from build123d import *

# Parameters (mm, degrees)
F0_W        = 50.8
F0_H        = 50.8
F1_DEPTH    = 546.1
F2_T        = -2.54
F3_T1_DEPTH = 506.0659394114
F5_D        = 41.275


# Not quite as in the source:
# - a fillet or chamfer that OpenCascade refuses, or shapes differently, is made with other operations: its cross-section is extruded or revolved along the edge and cut away or added


with BuildPart() as f1:
    # F0 (on Front) → F1 (new body, symmetric)
    with BuildSketch(Plane.XZ):
        Rectangle(F0_W, F0_H)
    extrude(amount=F1_DEPTH, both=True)

    # F2
    f2_openings = [f1.faces().sort_by_distance(p)[0] for p in [
        (0, -546.1, 0),
        (0, 546.1, 0),
    ]]
    offset(amount=F2_T, openings=f2_openings)

    # F3: chamfer of 50.8 x 87.9881810245 on 1 edges, made by hand

    # F3_s2 → F3_t1 (cut)
    with BuildSketch(Plane.XY.offset(-253.0329697057)):
        Polygon((25.4, 458.1118189755), (-25.4, 546.1), (25.4, 546.1), align=None)
    extrude(amount=F3_T1_DEPTH, mode=Mode.SUBTRACT)

    # F5 (through all)
    with Locations(Plane.XY.offset(25.4)):
        with Locations((0, -520.7)):
            Hole(F5_D / 2)


solid = f1.part
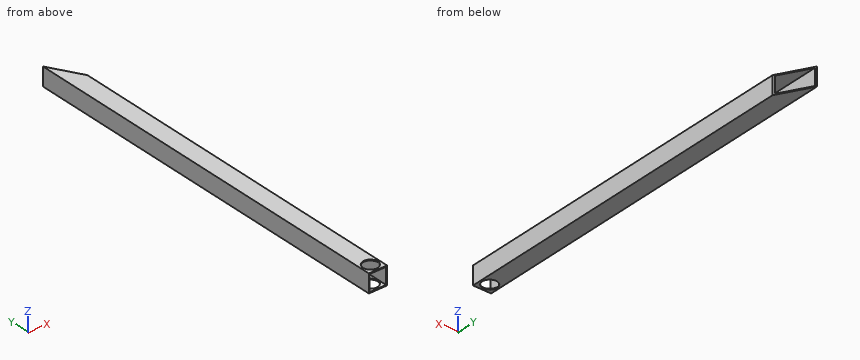
Geometry check sheet. Reference: the model listing, model coordinates, mm. Coordinates: 2 decimals unless noted, no trailing zeros. Order: outer loops, then holes, each group sorted by start corner. A loop starts at its lowest first (then second) coordinate and runs counter-clockwise, first axis right, second up. Notation, with made-up numbers: (-37, -6) - (-23, -6) arc R8 cw to (-23, 0) - close; hole circle Ø5 at (5, -13.5). An arc over 180 degrees is marked (long way). One line per item, written item: value.
(1) Sectioned sample at D-D (y = -156.5). Enter the section's corners in (x, z).
Data:
outline: (-25.4, -25.4) - (25.4, -25.4) - (25.4, 25.4) - (-25.4, 25.4) - close; hole (-22.86, -22.86) - (22.86, -22.86) - (22.86, 22.86) - (-22.86, 22.86) - close
(2) Sectioned sample at A-A (y = -520.7). Enter the section's corners in (x, z).
Data:
outline: (-25.4, -25.4) - (-20.64, -25.4) - (-20.64, -22.86) - (-22.86, -22.86) - (-22.86, 22.86) - (-20.64, 22.86) - (-20.64, 25.4) - (-25.4, 25.4) - close; (20.64, -25.4) - (25.4, -25.4) - (25.4, 25.4) - (20.64, 25.4) - (20.64, 22.86) - (22.86, 22.86) - (22.86, -22.86) - (20.64, -22.86) - close
(3) Sectioned sample at B-B (z = 5). Enter the section's corners in (x, y).
Data:
outline: (-25.4, -546.1) - (-22.86, -546.1) - (-22.86, 541.7) - (-25.4, 546.1) - close; (22.86, -546.1) - (25.4, -546.1) - (25.4, 458.11) - (22.86, 462.51) - close
(4) Sectioned sample at C-C (x = 0). Enter the section's corners in (y, z).
Data:
outline: (-546.1, -25.4) - (-541.34, -25.4) - (-541.34, -22.86) - (-546.1, -22.86) - close; (-546.1, 22.86) - (-541.34, 22.86) - (-541.34, 25.4) - (-546.1, 25.4) - close; (-500.06, -25.4) - (502.11, -25.4) - (502.11, -22.86) - (-500.06, -22.86) - close; (-500.06, 22.86) - (502.11, 22.86) - (502.11, 25.4) - (-500.06, 25.4) - close
(5) Thickness scan on probe 1 along Z at (x, y) = (-3, -147.5); probe 2 along X at (y, z) = (488.5, 2.5). Record the ranges inside material, lowest first. Write a range as from..to.
Data:
probe 1: z = -25.4..-22.86, 22.86..25.4
probe 2: x = -25.4..-22.86
